Build history of the part. All positions in model axes, mm. A direction names the side the tool comes from. Round coordinates to 2 decimals unless told otherwise and drop trailing zeros. Order: outer loops, then holes, each group sorted by start corner. A loop starts at its lowest first (then second) coordinate and runs counter-clockwise, first axis right, second up. Notation, with made-up numbers: M 5,1.25 L 28,1.25 A18 cw 28,12.25 Z; hole C -30.5,23 d5. An arc over 180 degrees is marked long. One line per item, written item: value. Start each with the question number.
Item 1: Pin check, flat tips, straight feed: pin 1 (1.7 mm diameter, centred on y = 25.5, z = 3.5, fed in from +X); pin 2 (2.5 mm diameter, centred on y = -25, z = 4, fed in from +X); pin 3 (1.9 mm diameter, centred on x = -149, z = 3.5, fed in from +Y). Stop position of each tip, or through.
Item 2: Band-saw the part on B-B, the plane x = 15.5. Write the cut outline in (y, z) (3 decimals).
Item 3: Probe L1, parallel to Y at x = 15.5, z = 3.5 (3 decimals); L2, parallel to Y at x = -133, z = 4.25 (3 decimals); L3, parallel to Y at x = 0, z = 4 (3 decimals). List the from-to ranges inside material, lowest first.
Item 4: Two-plate mould, pull along Y, no slides. Class faces 6 (the flat face through (-145.574, 16, 3)), 7 (the flat face through (-149, -12.7, 3)), 8 (the cylindrical face through (-2.38, 10.74, 3.13)): +Y half, -Y half, draft (parallel to the pull), parting line (faces both ways), or undercut.
Item 5: Band-saw the part on A-A, the plane y = -15.5. Write the cut outline in (x, z) (3 decimals).
Item 6: Band-saw the part on C-C, the plane y = 4.5. Write the cut outline in (x, z) (3 decimals).
Item 7: Band-saw the part on D-D, the plane y = -6. Write the cut outline in (x, z) (3 decimals).
Item 8: Tool access for faces 1 (the flat face through (-145.574, -17, 3)), 2 (the flat face through (-151.924, 0, 3)), 3 (the flat face through (-145.574, 26, 3)), 4 (the flat face through (-63, 0, 6.35)), 5 (the flat face through (-135, 24.079, 3)): list every direction of +Z, -Z, +X, -X, +Y, -Y with a clear straight run to the whole face (end or side of a thin tool).
Autodesk Inventor part; units mm, degrees
ref_plane "YZ Plane" through (0, 0, 0) normal (1, 0, 0) x (0, 1, 0)
ref_plane "XZ Plane" through (0, 0, 0) normal (0, 1, 0) x (-1, 0, 0)
ref_plane "XY Plane" through (0, 0, 0) normal (0, 0, 1) x (1, 0, 0)
sketch "Sketch1" plane through (0, 0, 0) normal (0, 0, 1) x (1, 0, 0)
  circle A0 centre (15.5, -15.5) radius 2
  circle A1 centre (-15.5, -15.5) radius 2
  circle A2 centre (15.5, 15.5) radius 2
  circle A3 centre (-15.5, 15.5) radius 2
  line L0 (-21.15, 15.4985) -> (-15.4985, 21.15)
  line L1 (-15.4985, 21.15) -> (15.4985, 21.15)
  line L2 (15.4985, 21.15) -> (21.15, 15.4985)
  line L3 (21.15, 15.4985) -> (21.15, -15.4985)
  line L4 (21.15, -15.4985) -> (15.4985, -21.15)
  line L5 (15.4985, -21.15) -> (-15.4985, -21.15)
  line L6 (-15.4985, -21.15) -> (-21.15, -15.4985)
  line L7 (-21.15, -15.4985) -> (-21.15, 15.4985)
  line L8 (28.575, -18.574) -> (28.575, 18.574)
  line L9 (28.575, 18.574) -> (18.574, 28.575)
  line L10 (18.574, 28.575) -> (-18.574, 28.575)
  line L11 (-18.574, 28.575) -> (-28.575, 18.574)
  line L12 (-28.575, 18.574) -> (-28.575, -18.574)
  line L13 (-28.575, -18.574) -> (-18.574, -28.575)
  line L14 (-18.574, -28.575) -> (18.574, -28.575)
  line L15 (18.574, -28.575) -> (28.575, -18.574)
  line L16 (-18.574, -28.575) -> (-145.574, -28.575)
  line L17 (-145.574, -28.575) -> (-145.574, 28.575)
  line L18 (-145.574, 28.575) -> (-18.574, 28.575)
  line L19 (-18.574, 28.575) -> (-18.574, -28.575)
  circle A4 centre (0, 0) radius 11
  dimension "d0" = 127
  dimension "d1" = 57.15
  dimension "d2" = 57.15
extrude "Extrusion1" add sketch "Sketch1" along normal blind 6.35
sketch "Sketch2" plane through (0, 0, 6.35) normal (0, 0, 1) x (1, 0, 0)
  line L0 (-130.4486, -16.3493) -> (-130.4486, -9.9993)
  line L1 (-126.7402, -9.9993) -> (-126.7402, -16.3493)
  line L2 (-130.4486, 9.0507) -> (-130.4486, 15.4007)
  line L3 (-126.7402, 15.4007) -> (-126.7402, 9.0507)
  line L4 (-126.7402, 12.7) -> (-130.4486, 12.7) construction
  line L5 (-126.7402, -12.7) -> (-130.9009, -12.7) construction
  circle A0 centre (-128.5944, 12.065) radius 1.8542
  circle A1 centre (-128.5944, -12.065) radius 1.8542
extrude "Extrusion2" cut sketch "Sketch2" against normal through all
sketch "Sketch3" plane through (0, 0, 6.35) normal (0, 0, 1) x (1, 0, 0)
  line L0 (-145.574, -28.575) -> (-145.574, 28.575)
  line L1 (-151.924, 20.3708) -> (-151.924, 24.0792)
  line L2 (-151.924, -24.5535) -> (-151.924, -20.8451)
  line L3 (-131.1543, 22.225) -> (-145.574, 22.225) construction
  line L4 (-131.1543, -22.225) -> (-145.574, -22.225) construction
  line L5 (-145.574, -20.3708) -> (-132.874, -20.3708)
  line L6 (-132.874, -20.3708) -> (-132.874, -24.0792)
  line L7 (-132.874, -24.0792) -> (-145.574, -24.0792)
  line L8 (-145.574, -24.0792) -> (-145.574, -20.3708)
  line L9 (-145.574, 24.0792) -> (-132.874, 24.0792)
  line L10 (-132.874, 24.0792) -> (-132.874, 20.3708)
  line L11 (-132.874, 20.3708) -> (-145.574, 20.3708)
  line L12 (-145.574, 20.3708) -> (-145.574, 24.0792)
  line L13 (-136.43, 26.162) -> (-139.224, 26.162)
  line L14 (-139.224, 26.162) -> (-139.224, 18.288)
  line L15 (-139.224, 18.288) -> (-136.43, 18.288)
  line L16 (-136.43, 18.288) -> (-136.43, 26.162)
  line L17 (-136.43, -18.288) -> (-139.224, -18.288)
  line L18 (-139.224, -18.288) -> (-139.224, -26.162)
  line L19 (-139.224, -26.162) -> (-136.43, -26.162)
  line L20 (-136.43, -26.162) -> (-136.43, -18.288)
  dimension "d9" = 12.7
  dimension "d10" = 2.794
  dimension "d11" = 7.874
  dimension "d12" = 3.937
  dimension "d13" = 3.937
  dimension "d14" = 7.874
  dimension "d15" = 3.937
  dimension "d16" = 3.937
  dimension "d17" = 6.35
  dimension "d18" = 6.35
  dimension "d19" = 2.794
extrude "Extrusion3" cut sketch "Sketch3" against normal through all
sketch "Sketch4" plane through (-145.574, -20.3708, 0) normal (-1, 0, 0) x (0, 0, 1)
  line L0 (6.35, 33.0708) -> (6.35, 7.6708)
  line L1 (6.35, 7.6708) -> (0, 7.6708)
  line L2 (0, 7.6708) -> (0, 33.0708)
  line L3 (0, 33.0708) -> (6.35, 33.0708)
  point P0 (0, 20.3708)
extrude "Extrusion4" add sketch "Sketch4" along normal blind 6.35
equation "\"d2\" = d1"
equation "\"d12\" = d13"
equation "\"d15\" = d16"
properties part number "tiltColumnNonStepperSide02_RB01" material "Titanium"
Output:
1. pin 1: stops at x = 22.5
1. pin 2: stops at x = 23.4
1. pin 3: stops at y = 12.7
2. outline: M -28.575,0 L -17.5,0 L -17.5,6.35 L -28.575,6.35 Z; M -13.5,0 L 13.5,0 L 13.5,6.35 L -13.5,6.35 Z; M 17.5,0 L 28.575,0 L 28.575,6.35 L 17.5,6.35 Z
3. L1: y = -28.575 to -17.5, -13.5 to 13.5, 17.5 to 28.575
3. L2: y = -28.575 to -24.079, -20.371 to 20.371, 24.079 to 28.575
3. L3: y = -28.575 to -11, 11 to 28.575
4. face 6: draft
4. face 7: -Y half
4. face 8: undercut
5. outline: M -145.574,0 L -17.5,0 L -17.5,6.35 L -145.574,6.35 Z; M -13.5,0 L 13.5,0 L 13.5,6.35 L -13.5,6.35 Z; M 17.5,0 L 28.575,0 L 28.575,6.35 L 17.5,6.35 Z
6. outline: M -151.924,0 L -10.037,0 L -10.037,6.35 L -151.924,6.35 Z; M 10.037,0 L 28.575,0 L 28.575,6.35 L 10.037,6.35 Z
7. outline: M -151.924,0 L -9.22,0 L -9.22,6.35 L -151.924,6.35 Z; M 9.22,0 L 28.575,0 L 28.575,6.35 L 9.22,6.35 Z
8. face 1: +Z, -Z, -X, -Y
8. face 2: +Z, -Z, -X, +Y, -Y
8. face 3: +Z, -Z, -X, +Y
8. face 4: +Z, +X, -X, +Y, -Y
8. face 5: +Z, -Z, -X
